Geometry: see drawing. Coordinates: mm, zero at the bounding-box minimum. Coordinates: 2 decimals unless noted, no trailing zeros. Write each loop counter-clockwise with the first axis right and the second up, starting at its lowest first coordinate (ties: lowest second). Pieces come first, ordered by that corner, then holes. Notation, with made-up numbers: (-12, 80.25) -> (30, 80.25) arc R12 ccw to (30, 94.25) -> close; hole circle Ø5 at (-36.5, -17.5). An arc over 180 degrees is marked (long way). Answer as a JSON object with one key per item and string values. Group by question number.
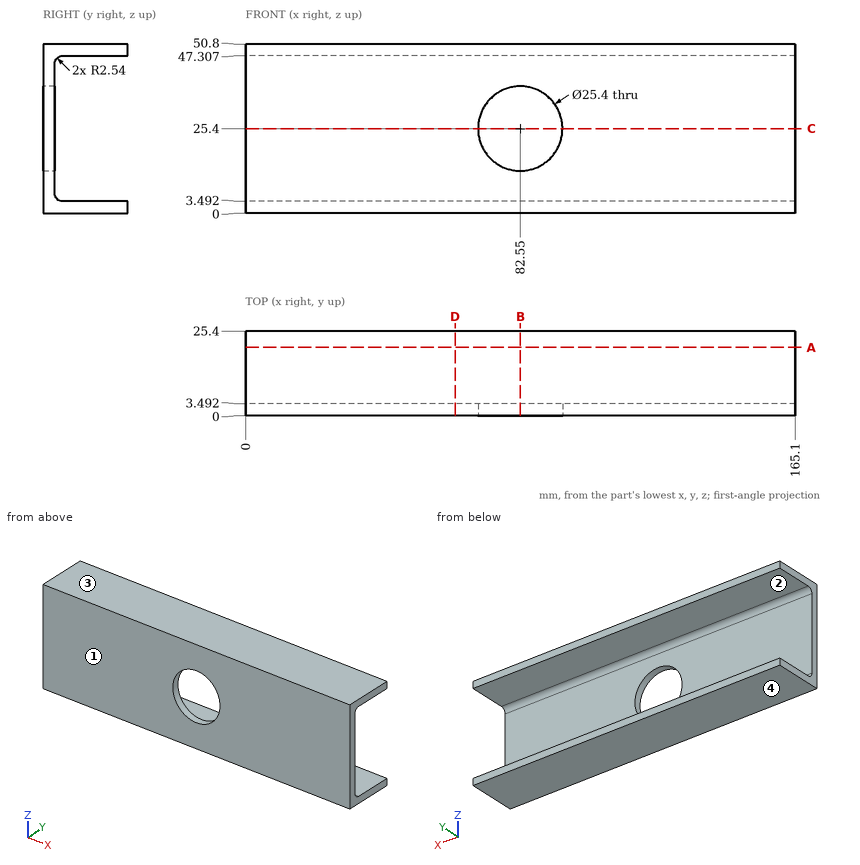
Item 1: Mould query, pull axis Z, two halves, no side actions, for the marked faces 1, 2, 3 and 4. Classes: +Z half, -Z half, draft (parallel to the pull), parting line (faces both ways), or undercut.
Item 2: Section C-C on z = 25.4. Output: boundary loops of the cut face in (x, y), then the cut area to 3 significant figures.
Item 3: Section B-B on x = 82.55. Output: boundary loops of the cut face in (y, z).
Item 4: Section A-A on y = 20.5. Output: boundary loops of the cut face in (x, z), then the cut area to 3 significant figures.
Item 5: Ray query, L1, parallel to X at y = 2.05, z = 25.4; L2, parallel to Z at x = 95.5, y = 16.5; L3, parallel to Y at x = 85.5, z = 43. Return the intervals inside material, ascending. Write a range as [from, to].
Item 6: Contact query for flat-ended pins moving along their axis: pin 1 (23 mm diameter, centred on x = 82.55, z = 25.4, fed in from -Y); pin 2 (1.5 mm diameter, centred on x = 144, z = 44.5, fed in from +Y). Output: stop coordinate, or through.
Item 7: Section D-D on x = 63. Output: boundary loops of the cut face in (y, z).
Answer sheet:
{
 "1": {"face 1": "draft", "face 2": "undercut", "face 3": "+Z half", "face 4": "-Z half"},
 "2": {"outline": "(0, 0) -> (69.85, 0) -> (69.85, 3.49) -> (0, 3.49) -> close; (95.25, 0) -> (165.1, 0) -> (165.1, 3.49) -> (95.25, 3.49) -> close", "area": "488 mm^2"},
 "3": {"outline": "(0, 0) -> (25.4, 0) -> (25.4, 3.49) -> (6.03, 3.49) arc R2.54 cw to (3.49, 6.03) -> (3.49, 12.7) -> (0, 12.7) -> close; (0, 38.1) -> (3.49, 38.1) -> (3.49, 44.77) arc R2.54 cw to (6.03, 47.31) -> (25.4, 47.31) -> (25.4, 50.8) -> (0, 50.8) -> close"},
 "4": {"outline": "(0, 0) -> (165.1, 0) -> (165.1, 3.49) -> (0, 3.49) -> close; (0, 47.31) -> (165.1, 47.31) -> (165.1, 50.8) -> (0, 50.8) -> close", "area": "1,150 mm^2"},
 "5": {"L1": "x = [0, 69.85], [95.25, 165.1]", "L2": "z = [0, 3.49], [47.31, 50.8]", "L3": "y = [0, 3.49]"},
 "6": {"pin 1": "passes through", "pin 2": "stops at y = 3.54"},
 "7": {"outline": "(0, 0) -> (25.4, 0) -> (25.4, 3.49) -> (6.03, 3.49) arc R2.54 cw to (3.49, 6.03) -> (3.49, 44.77) arc R2.54 cw to (6.03, 47.31) -> (25.4, 47.31) -> (25.4, 50.8) -> (0, 50.8) -> close"}
}
